For this review, take the finished solid that the model builds, in its own axes (mm). Give positions to 0.01 mm unless a question says otherwise; leave off trailing zeros. Order: outer loops, then holes, each group sorted by start corner. A loop starts at its lowest first (then second) coordinate and runs counter-clockwise, first axis right, second up. Notation, with made-up numbers: (-32, 30.5) - (14, 30.5) arc R20 ccw to (14, 52.5) - close; hole circle Ø6 at (39.25, -28). An arc over 180 degrees is marked (long way). Answer as a JSON object with one key per item and string values. Group by question number.
from build123d import *

# Parameters (mm, degrees)
ESQUISSE1_W        = 20
ESQUISSE1_H        = 10
ESQUISSE1_R        = 1.25
BOSS_EXTRU_1_DEPTH = 7
CHANFREIN1_SIZE    = 2


with BuildPart() as part:
    # Esquisse1 → Boss.-Extru.1 (new body)
    with BuildSketch(Plane(origin=(0, 0, 0), x_dir=(1, 0, 0), z_dir=(0, 1, 0))):
        Rectangle(ESQUISSE1_W, ESQUISSE1_H)
        with Locations(Location((4.75, -2.6, 0), (0, 0, 270))):
            Circle(ESQUISSE1_R, mode=Mode.SUBTRACT)
        with Locations(Location((-4.75, -2.6, 0), (0, 0, 270))):
            Circle(ESQUISSE1_R, mode=Mode.SUBTRACT)
    extrude(amount=BOSS_EXTRU_1_DEPTH)

    # Chanfrein1
    chanfrein1_edges = [part.edges().sort_by_distance(p)[0] for p in [
        (10, 3.5, 5),
        (-10, 3.5, 5),
        (-10, 3.5, -5),
        (10, 3.5, -5),
    ]]
    chamfer(chanfrein1_edges, length=CHANFREIN1_SIZE)


solid = part.part
1) Mouldability with a two-part tool opening along X and no side actions: class faces 1 (the face through (3.53, 3.45, 2.33)), 2 (the face through (0, 3, -5)), 3 (the face through (-5.97, 3.45, 2.33)), 4 (the face through (9, 3, 4)) as released by +X, released by -X, zero draft, split by the parting line, or undercut.
2) For line 1 (X direction, y = 3.75, z = 2.6); line 2 (X direction, y = 1, z = 2.25); line 3 (Z direction, x = -5, y = 6.5), list the stretches that pass through material, from the lowest coordinate up.
3) Consider section A-A (x = -4.75). Give the boundary of the cut face in (y, z).
4) Consider section B-B (z = 2.6). Give the boundary of the cut face in (x, y).
5) Consider section C-C (y = 3.75). Give the boundary of the cut face in (x, z).
Result set:
{
 "1": {"face 1": "undercut", "face 2": "zero draft", "face 3": "undercut", "face 4": "released by +X"},
 "2": {"line 1": "x = -10 to -6, -3.5 to 3.5, 6 to 10", "line 2": "x = -10 to -5.95, -3.55 to 3.55, 5.95 to 10", "line 3": "z = -5 to 1.38, 3.82 to 5"},
 "3": {"outline": "(0, -5) - (7, -5) - (7, 1.35) - (0, 1.35) - close; (0, 3.85) - (7, 3.85) - (7, 5) - (0, 5) - close"},
 "4": {"outline": "(-10, 0) - (-6, 0) - (-6, 7) - (-10, 7) - close; (-3.5, 0) - (3.5, 0) - (3.5, 7) - (-3.5, 7) - close; (6, 0) - (10, 0) - (10, 7) - (6, 7) - close"},
 "5": {"outline": "(-10, -3) - (-8, -5) - (8, -5) - (10, -3) - (10, 3) - (8, 5) - (-8, 5) - (-10, 3) - close; hole circle Ø2.5 at (-4.75, 2.6); hole circle Ø2.5 at (4.75, 2.6)"}
}
